Autodesk Inventor part; units mm, degrees
ref_plane "YZ Plane" through (0, 0, 0) normal (1, 0, 0) x (0, 1, 0)
ref_plane "XZ Plane" through (0, 0, 0) normal (0, 1, 0) x (-1, 0, 0)
ref_plane "XY Plane" through (0, 0, 0) normal (0, 0, 1) x (1, 0, 0)
sketch "Sketch1" plane through (0, 0, 0) normal (0, 1, 0) x (-1, 0, 0)
  circle A0 centre (0, 262.5) radius 3 construction
  circle A1 centre (0, -262.5) radius 3 construction
  line L0 (-25, -300) -> (25, -300) construction
  line L1 (25, -300) -> (25, 300) construction
  line L2 (-25, 300) -> (25, 300) construction
  line L3 (-25, -300) -> (-25, 300) construction
  circle A2 centre (71, 10) radius 3
  circle A3 centre (71, -10) radius 3
  arc A4 (5.8119, -39.1259) -> (-27.7565, -64.4201) centre (-3.9972, -61.0298) ccw construction
  arc A5 (-27.7597, 64.3976) -> (5.8116, 39.1072) centre (-4, 61.01) ccw construction
  line L4 (71, 10) -> (71, -10) construction
  circle A6 centre (71, -10) radius 9 construction
  circle A7 centre (71, 10) radius 9 construction
  line L5 (80, 10) -> (80, -10)
  line L6 (25, 35) -> (73.8743, 18.5287)
  line L7 (25, 35) -> (-25, 35)
  line L8 (-25, 35) -> (-25, -35)
  line L9 (-25, -35) -> (25, -35)
  line L10 (25, -35) -> (25, 35) construction
  line L11 (25, 35) -> (-25, -35) construction
  line L12 (-25, 35) -> (25, -35) construction
  line L13 (25, -35) -> (73.8743, -18.5287)
  arc A8 (80, 10) -> (73.8743, 18.5287) centre (71, 10) ccw
  arc A9 (73.8743, -18.5287) -> (80, -10) centre (71, -10) ccw
  line L14 (25, 35) -> (25, -35)
  line L15 (15, -25) -> (-15, -25)
  line L16 (-15, -25) -> (-15, 25)
  line L17 (-15, 25) -> (15, 25)
  line L18 (15, 25) -> (15, -25)
  line L19 (25, 35) -> (73.8743, 18.5287)
  line L20 (73.8743, 18.5287) -> (70.0419, 7.1571)
  line L21 (70.0419, 7.1571) -> (21.1676, 23.6284)
  line L22 (21.1676, 23.6284) -> (25, 35)
  line L23 (25, -35) -> (73.8743, -18.5287)
  line L24 (73.8743, -18.5287) -> (70.0419, -7.1571)
  line L25 (70.0419, -7.1571) -> (21.1676, -23.6284)
  line L26 (21.1676, -23.6284) -> (25, -35)
  line L27 (62, 10) -> (62, -10)
  line L28 (-25, 35) -> (-16, 35) construction
  line L29 (-16, 35) -> (-16, -35) construction
  line L30 (-16, -35) -> (-25, -35) construction
  line L31 (-25, -35) -> (-25, 35) construction
  line L32 (25, 35) -> (16, 35) construction
  line L33 (16, 35) -> (16, -35) construction
  line L34 (16, -35) -> (25, -35) construction
  line L35 (25, -35) -> (25, 35) construction
  line L36 (-25, 35) -> (25, 35) construction
  line L37 (25, 35) -> (25, 30) construction
  line L38 (25, 30) -> (-25, 30) construction
  line L39 (-25, 30) -> (-25, 35) construction
  line L40 (-25, -35) -> (25, -35) construction
  line L41 (25, -35) -> (25, -30) construction
  line L42 (25, -30) -> (-25, -30) construction
  line L43 (-25, -30) -> (-25, -35) construction
  circle A10 centre (16, 30) radius 2.5
  circle A11 centre (16, -30) radius 2.5
  circle A12 centre (-16, -30) radius 2.5
  circle A13 centre (-16, 30) radius 2.5
  point P0 (0, 0)
  point P1 (62, -9.8673)
  point P2 (25, -22.3369)
  point P3 (25, 22.3369)
  point P4 (62, 9.8673)
  dimension "d0" = 18
  dimension "d1" = 18
  dimension "d2" = 70
  dimension "d3" = 10
  dimension "d4" = 12
  dimension "d5" = 12
  dimension "d6" = 9
  dimension "d7" = 9
  dimension "d8" = 5
  dimension "d9" = 5
  dimension "d10" = 5
  dimension "d11" = 5
  dimension "d12" = 5
  dimension "d13" = 5
extrude "Extrusion1" add sketch "Sketch1" along normal blind 5 contours L20 A2 | L21 L14 L6 L20 A2 | A2 L20 | A2 L20 A8 L5 A9 L24 A3 L25 L27 L21 | L21 L22 L14 | L14 L25 L26 L9 L8 L7 L22 L21 | L25 A3 L24 L13 L14 | L14 L26 L25 | L24 A3 | A3 L24
fillet "Fillet1" radius 5 8 edges at (-15, 2.5, -25) (-15, 2.5, 25) (15, 2.5, 25) (15, 2.5, -25) (-25, 2.5, -22.3369) (-25, 2.5, 22.3369) (-62, 2.5, -9.8673) (-62, 2.5, 9.8673)
fillet "Fillet2" radius 2 4 edges at (25, 2.5, -35) (25, 2.5, 35) (-25, 2.5, -35) (-25, 2.5, 35)
sketch "Sketch3" plane through (0, 5, 0) normal (0, 1, 0) x (1, 0, 0)
  arc A0 (-80, -10) -> (-73.8743, -18.5287) centre (-71, -10) ccw
  arc A1 (-73.8743, 18.5287) -> (-80, 10) centre (-71, 10) ccw
  point P0 (0, 0)
hole "Hole1" at (-71, 5, 10) at (-71, 5, -10) direction (0, -1, 0) diameter 6 end through all
properties part number "pistonMount"
Here's how the part is built. I have some questions about the finished solid (model axes, mm). A direction names the side the tool comes from. Give positions to 0.01 mm unless a question says otherwise; leave off trailing zeros. Loops run counter-clockwise (first coordinate to the right, second up) from the corner with the lowest first, then second, coordinate; pieces in that order, holes last. Notation, with made-up numbers: (67, -32.5) -> (115, -32.5) arc R5 ccw to (115, -23.5) -> close; hole circle Ø10 at (20, 60). An arc over 180 degrees is marked (long way). Answer as a JSON object with one key per item and string values. Group by question number.
Item 1: Imagine slicing it at A-A on x = 6. Write out the boundary of the cut face in (y, z).
Item 2: Imagine slicing it at C-C on y = 2. Give the number of separate pieces and of enclosed holes in the cut face, then the cut area to 3 significant figures.
Item 3: On a 3-axis mill with a long thin cutter (end or side, diameter ignored), from which of +Z, -Z, +X, -X, +Y, -Y can I reach the whole of each face in a straight line? I mean faces 4 (the flat face through (15, 2, 0)), 5 (the flat face through (25, 2, 0)). Say none if no direction works.
Item 4: Imagine slicing it at B-B on z = 22.5. Write out the boundary of the cut face in (x, y), then the cut area to 3 significant figures.
Item 5: Imagine slicing it at D-D on x = -71. Write out the boundary of the cut face in (y, z), then the cut area to 3 significant figures.
Item 6: I need wall thicknesses on L1, parallel to Z at x = 16, y = 2.8; L2, parallel to Z at x = -0.5, y = 0.3; L3, parallel to X at y = 0.85, z = -1.5. Which ranges of each line are inside material? Lowest first, please.
Item 7: Will this pin go through, and if not, where does the flat tip stop? pin 1 (4 mm diameter, centred on x = -16, z = -30, fed in from -Y).
Item 8: Thinking about a two-plate mould opening in Z: for faces 1 (the flat face through (-27, 0, -23)), 2 (the cylindrical face through (24.4, 2.54, 34.43)), 3 (the flat face through (-25, 2, 0)), which applies, pulls with the +Z half, pulls with the -Z half, needs draft (parallel to the pull), parting line crosses it, or undercut?
Answer list:
{
 "1": {"outline": "(0, -35) -> (5, -35) -> (5, -25) -> (0, -25) -> close; (0, 25) -> (5, 25) -> (5, 35) -> (0, 35) -> close"},
 "2": {"separate pieces": "1", "enclosed holes": "8", "area": "3,540 mm2"},
 "3": {"face 4": "+Y, -Y", "face 5": "+Z, -Z, +X, +Y, -Y"},
 "4": {"outline": "(-62.09, 0) -> (-14.33, 0) -> (-14.33, 5) -> (-62.09, 5) -> close; (14.33, 0) -> (25, 0) -> (25, 5) -> (14.33, 5) -> close", "area": "292 mm2"},
 "5": {"outline": "(0, -19.5) -> (5, -19.5) -> (5, -13) -> (0, -13) -> close; (0, -7) -> (5, -7) -> (5, 7) -> (0, 7) -> close; (0, 13) -> (5, 13) -> (5, 19.5) -> (0, 19.5) -> close", "area": "135 mm2"},
 "6": {"L1": "z = -35 to -32.5, -27.5 to 27.5, 32.5 to 35", "L2": "z = -35 to -25, 25 to 35", "L3": "x = -80 to -62, -25 to -15, 15 to 25"},
 "7": {"pin 1": "passes through"},
 "8": {"face 1": "needs draft", "face 2": "pulls with the +Z half", "face 3": "undercut"}
}
